The listing builds one solid part. Answer for the finished solid, in the listing's coordinates (mm). Face numbers are marked on the shaded views. A direction names the side the tool comes from. Coordinates: 2 decimals unless noted, no trailing zeros. Order: outer loops, then holes, each group sorted by start corner. A loop starts at its lowest first (then second) coordinate and runs counter-clockwise, first axis right, second up.
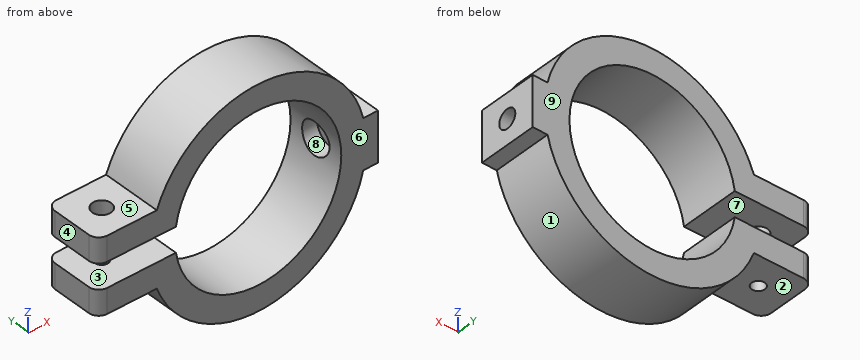
Autodesk Inventor part; units mm, degrees
ref_plane "Work Plane3" through (19.75, 0, 0) normal (1, 0, 0) x (0, 1, 0)
ref_plane "XZ Plane" through (0, 0, 0) normal (0, 1, 0) x (-1, 0, 0)
ref_plane "XY Plane" through (0, 0, 0) normal (0, 0, 1) x (1, 0, 0)
sketch "Sketch1" plane through (0, 0, 0) normal (0, 1, 0) x (-1, 0, 0)
  arc A0 (16.5624, 2.5) -> (16.5624, -2.5) centre (0, 0) ccw
  arc A1 (20.416, 7.5) -> (20.416, -7.5) centre (0, 0) ccw
  line L0 (32.416, 7.5) -> (20.416, 7.5)
  line L1 (16.5624, 2.5) -> (32.416, 2.5)
  line L2 (32.416, 2.5) -> (32.416, 7.5)
  line L3 (32.416, -2.5) -> (16.5624, -2.5)
  line L4 (20.416, -7.5) -> (32.416, -7.5)
  line L5 (32.416, -7.5) -> (32.416, -2.5)
  line L6 (26.416, 5) -> (26.416, -5) construction
  line L7 (-21.1675, -5) -> (-24.1675, -5)
  line L8 (-24.1675, -5) -> (-24.1675, 5)
  line L9 (-24.1675, 5) -> (-21.1675, 5)
  line L10 (-21.1675, 5) -> (-21.1675, -5)
  point P0 (32.416, 5)
  point P1 (32.416, -5)
  point P2 (26.416, 0)
  point P3 (26.416, -7.5)
  point P4 (-16.75, 0)
  point P5 (-24.1675, 0)
  dimension "d0" = 33.5
  dimension "d1" = 5
  dimension "d4" = 5
  dimension "d5" = 5
  dimension "d6" = 10
  dimension "d7" = 12
  dimension "d35" = 10
  dimension "d36" = 3
extrude "Extrusion1" add sketch "Sketch1" along normal mid plane 12
sketch "Sketch2" plane through (-32.416, 6, 7.5) normal (0, 0, 1) x (1, 0, 0)
  line L0 (0, 0) -> (0, -12)
  line L1 (0, 0) -> (12, 0)
  point P0 (32.416, -6)
  point P1 (6, -6)
  point P2 (0, -6)
  point P3 (6, 0)
hole "Hole1" at (-26.416, 0, 7.5) direction (0, 0, -1) diameter 3.797 depth 5
sketch "Sketch3" plane through (-20.416, 6, -7.5) normal (0, 0, -1) x (-1, 0, 0)
  line L0 (8.3161, -1.9884) -> (10.6322, -6)
  line L1 (10.6322, -6) -> (8.3161, -10.0116)
  line L2 (8.3161, -10.0116) -> (3.6839, -10.0116)
  line L3 (3.6839, -10.0116) -> (1.3678, -6)
  line L4 (1.3678, -6) -> (3.6839, -1.9884)
  line L5 (3.6839, -1.9884) -> (8.3161, -1.9884)
  circle A0 centre (6, -6) radius 1.8985
  point P0 (-20.416, -6)
  dimension "d17" = 8.0232
extrude "Extrusion2" [suppressed]
fillet "Fillet1" radius 2 4 edges at (-32.416, -6, -5) (-32.416, 6, -5) (-32.416, 6, 5) (-32.416, -6, 5)
ref_plane "Work Plane3" through (19.75, 0, 0) normal (1, 0, 0) x (0, 1, 0)
sketch "Sketch5" plane through (19.75, 0, 0) normal (1, 0, 0) x (0, 1, 0)
  circle A0 centre (0, 0) radius 3.25
  dimension "d25" = 6.5
extrude "Extrusion4" cut sketch "Sketch5" against normal up to next
hole "Hole2" at (19.75, 0, 0) direction (1, 0, 0) diameter 3.797 end through all
sketch "Sketch6" plane through (-20.416, -6, -7.5) normal (0, 0, -1) x (-1, 0, 0)
  line L0 (10, 0) -> (-3.8536, 0)
  point P0 (-20.416, 6)
  point P1 (6, 6)
hole "Hole3" at (-26.416, 0, -7.5) direction (0, 0, 1) diameter 2.642 depth 5
equation "\"d5\" = d4"
properties part number "CameraClamp"
(1) Find section A-A (y = 0). Give the number of separate pieces and of enclosed holes in the cut face, and give its area (3 significant figures).
(2) Find section B-B (z = 0). Write down the section's boundary in (x, y).
(3) Each of these flat-tipped pins is pushed along its axis until it touches: pin 1 Ø4 at (x, y) = (2.5, 0) entering from +Z; pin 2 Ø6 at (x, y) = (-23.5, -2) entering from +Z; pin 3 Ø3 at (x, y) = (-22.5, 1.5) entering from -Z. Where does it stop, or does it pass through?
(4) The mould has two halves that part along Y. Classify the marked faces 6, 7, 8 and 9: released by +Y, released by -Y, zero draft, split by the parting line, or undercut.
(5) Find section C-C (x = 0). Write down the section's boundary in (y, z).
(6) For the marked faces 1, 2, 3, 4 and 5, determine the directions among +Z, -Z, +X, -X, +Y, -Y from which every point of the face is accessible in a straight line to the end or side of a thin tool.
(7) Find section D-D (z = 6.5). Write down the section's boundary in (x, y).
(8) Consider line 1 (Y direction, x = 19.05, z = 0); line 2 (X direction, y = -0.25, z = -7); line 3 (Z direction, x = 0.5, y = -2.75). Determine where each line is inside the solid, lowest interval first.
Findings below:
1. separate pieces: 4
1. enclosed holes: 0
1. area: 650 mm2
2. outline: (16.75, -6) - (24.17, -6) - (24.17, -1.9) - (19.75, -1.9) - (19.75, -3.25) - (16.75, -3.25) - close; (16.75, 3.25) - (19.75, 3.25) - (19.75, 1.9) - (24.17, 1.9) - (24.17, 6) - (16.75, 6) - close
3. pin 1: stops at z = 21.74
3. pin 2: stops at z = 7.5
3. pin 3: stops at z = -7.5
4. face 6: released by -Y
4. face 7: zero draft
4. face 8: undercut
4. face 9: released by +Y
5. outline: (-6, -21.75) - (6, -21.75) - (6, -16.75) - (-6, -16.75) - close; (-6, 16.75) - (6, 16.75) - (6, 21.75) - (-6, 21.75) - close
6. face 1: -Z, +Y, -Y
6. face 2: -Z, -X, +Y, -Y
6. face 3: -X, +Y, -Y
6. face 4: +Z, -Z, -X, +Y, -Y
6. face 5: +Z, -X, +Y, -Y
7. outline: (-32.42, -4) arc R2 ccw to (-30.42, -6) - (-15.44, -6) - (-15.44, 6) - (-30.42, 6) arc R2 ccw to (-32.42, 4) - close; (15.44, -6) - (20.76, -6) - (20.76, 6) - (15.44, 6) - close; hole circle Ø3.8 at (-26.42, 0)
8. line 1: y = -6 to -3.25, 3.25 to 6
8. line 2: x = -32.42 to -27.71, -25.12 to -15.22, 15.22 to 20.59
8. line 3: z = -21.74 to -16.74, 16.74 to 21.74
